The model under review builds one solid part; all positions refer to its coordinate system, in mm. Give positions to 0.01 mm unless a question says otherwise; leave off trailing zeros. Loops run counter-clockwise (first coordinate to the right, second up) from the corner with the lowest first, then second, coordinate; pieces in that order, holes last. Notation, with made-up numbers: M 46,66.5 L 92,66.5 A23 cw 92,105.5 Z; hole C 5.5,-26 d6. An arc over 180 degrees is marked long. Write item = value, one per line. Start each with the question number.
1. For pin 1 (22 mm diameter, centred on x = -101.6, z = 44.45, fed in from +Y); pin 2 (15 mm diameter, centred on x = -101.6, z = -44.45, fed in from +Y), all flat-tipped, find the tip position at first contact; note any pin that passes through.
2. We need section A-A on z = -44.45. Give the boundary of the cut face in (x, y) (3 decimals), then the cut area to 3 significant figures.
3. Wall thickness on line 1 along Z through (x, y) = (-101.6, -3.75) (3 decimals); line 2 along X through (y, z) = (-3, 44.45) (3 decimals); line 3 along Z through (x, y) = (-139.7, -4) (3 decimals): over which ranges is each line inside the solid? List them lowest first. Write a range as from..to.
4. We need section C-C on y = -2.5. Give the boundary of the cut face in (x, z) (3 decimals), then the cut area to 3 significant figures.
5. We need section B-B on x = -101.6. Give the boundary of the cut face in (y, z) (3 decimals), then the cut area to 3 significant figures.
from build123d import *

# Parameters (mm, degrees)
F0_W     = 304.8
F0_H     = 139.7
F1_DEPTH = 6.35
F3_D     = 19.05


with BuildPart() as f1:
    # F0 (on Front) → F1 (new body)
    with BuildSketch(Plane.XZ):
        Rectangle(F0_W, F0_H)
    extrude(amount=F1_DEPTH)

    # F3 (through all)
    with Locations(Plane(origin=(0, 0, 0), x_dir=(1, 0, 0), z_dir=(0, 1, 0))):
        with Locations((-101.6, 44.45), (-139.7, 0), (-101.6, -44.45)):
            Hole(F3_D / 2)


solid = f1.part
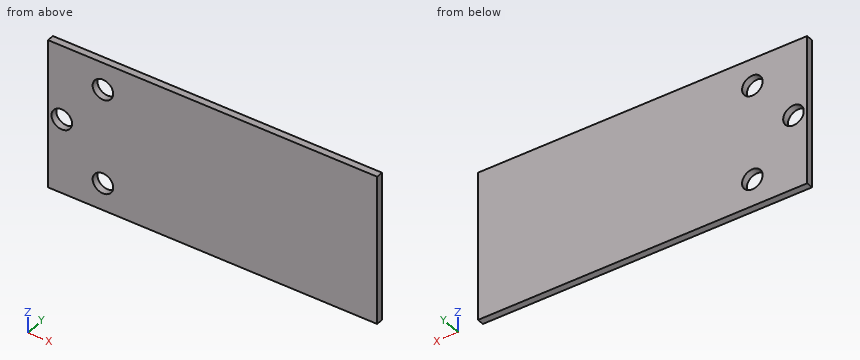
Final values:
q1.pin_1 = 0
q1.pin_2 = through
q2.outline = M -152.4,-6.35 L -111.125,-6.35 L -111.125,0 L -152.4,0 Z; M -92.075,-6.35 L 152.4,-6.35 L 152.4,0 L -92.075,0 Z
q2.area = 1,810 mm²
q3.line_1 = -69.85..-53.975, -34.925..34.925, 53.975..69.85
q3.line_2 = -152.4..-111.125, -92.075..152.4
q3.line_3 = -69.85..-9.525, 9.525..69.85
q4.outline = M -152.4,-69.85 L 152.4,-69.85 L 152.4,69.85 L -152.4,69.85 Z; hole C -139.7,0 d19.05; hole C -101.6,-44.45 d19.05; hole C -101.6,44.45 d19.05
q4.area = 41,700 mm²
q5.outline = M -6.35,-69.85 L 0,-69.85 L 0,-53.975 L -6.35,-53.975 Z; M -6.35,-34.925 L 0,-34.925 L 0,34.925 L -6.35,34.925 Z; M -6.35,53.975 L 0,53.975 L 0,69.85 L -6.35,69.85 Z
q5.area = 645 mm²
